Geometry: final body of the model. Coordinates: model frame, mm. A direction names the side the tool comes from. Give positions to 0.01 mm unless a question says otherwise; leave off trailing zeros. Order: outer loops, then holes, each group sorted by start corner. A loop starts at its lowest first (then second) coordinate and runs counter-clockwise, first axis right, second up. Notation, with made-up numbers: (-26, 75.5) -> (18, 75.5) arc R20 ccw to (18, 99.5) -> close; hole circle Ø9 at (-35, -34.5). An arc over 180 degrees is marked (long way). Write item = value, one per line.
```python
from build123d import *

# Parameters (mm, degrees)
F0_W     = 11
F0_H     = 30
F1_DEPTH = 24
F3_DEPTH = 11
F4_R     = 5
F4_R_2   = 2.5
F5_DEPTH = 41.001
F6_R     = 13
F7_R     = 5
F8_R     = 2


with BuildPart() as f1:
    # F0 (on Right) → F1 (new body, symmetric)
    with BuildSketch(Plane.YZ):
        with BuildLine():
            Line((-56, 0), (-30, 0))
            ThreePointArc((-30, 0), (-29.4730143031, 5.5983415304), (-27.9105714739, 11))
            Line((-27.9105714739, 11), (-56, 11))
            Line((-56, 11), (-56, 0))
        make_face()
        with BuildLine():
            Line((-30, 0), (-19, 0))
            ThreePointArc((-19, 0), (-18.1017503893, 5.7729223833), (-15.4919333848, 11))
            Line((-15.4919333848, 11), (-27.9105714739, 11))
            ThreePointArc((-27.9105714739, 11), (-29.4730143031, 5.5983415304), (-30, 0))
        make_face()
        with BuildLine():
            ThreePointArc((15.4919333848, 11), (18.1017503893, 5.7729223833), (19, 0))
            Line((19, 0), (30, 0))
            ThreePointArc((30, 0), (29.4730143031, 5.5983415304), (27.9105714739, 11))
            Line((27.9105714739, 11), (15.4919333848, 11))
        make_face()
        with BuildLine():
            ThreePointArc((-15.4919333848, 11), (0, 19), (15.4919333848, 11))
            Line((15.4919333848, 11), (27.9105714739, 11))
            ThreePointArc((27.9105714739, 11), (0, 30), (-27.9105714739, 11))
            Line((-27.9105714739, 11), (-15.4919333848, 11))
        make_face()
        with BuildLine():
            ThreePointArc((27.9105714739, 11), (29.4730143031, 5.5983415304), (30, 0))
            Line((30, 0), (51, 0))
            Line((51, 0), (51, 11))
            Line((51, 11), (40, 11))
            Line((40, 11), (27.9105714739, 11))
        make_face()
        with Locations((45.5, 26)):
            Rectangle(F0_W, F0_H)
    extrude(amount=F1_DEPTH, both=True)

    # F2 (on face) → F3 (cut, through all)
    with BuildSketch(Plane(origin=(0, 51, 0), x_dir=(-1, 0, 0), z_dir=(0, 1, 0))):
        with BuildLine():
            ThreePointArc((-6.5, 25), (0, 31.5), (6.5, 25))
            Line((6.5, 25), (6.5, 41))
            Line((6.5, 41), (-6.5, 41))
            Line((-6.5, 41), (-6.5, 25))
        make_face()
        with BuildLine():
            ThreePointArc((-6.5, 25), (0, 18.5), (6.5, 25))
            ThreePointArc((6.5, 25), (0, 31.5), (-6.5, 25))
        make_face()
    extrude(amount=-F3_DEPTH, mode=Mode.SUBTRACT)

    # F4 (on face) → F5 (cut, through all)
    with BuildSketch(Plane(origin=(0, 0, 0), x_dir=(1, 0, 0), z_dir=(0, 0, -1))):
        with Locations((11, 37.5)):
            Circle(F4_R)
        Circle(F4_R_2)
        with Locations((-11, 37.5)):
            Circle(F4_R)
    extrude(amount=-F5_DEPTH, mode=Mode.SUBTRACT)

    # F6
    f6_edges = [f1.edges().sort_by_distance(p)[0] for p in [
        (-24, -56, 5.5),
        (24, -56, 5.5),
    ]]
    fillet(f6_edges, radius=F6_R)

    # F7
    f7_edges = [f1.edges().sort_by_distance(p)[0] for p in [
        (-24, 45.5, 41),
        (24, 45.5, 41),
    ]]
    fillet(f7_edges, radius=F7_R)

    # F8
    f8_edges = [f1.edges().sort_by_distance(p)[0] for p in [
        (0, -27.910571, 11),
        (0, 27.910571, 11),
    ]]
    fillet(f8_edges, radius=F8_R)


solid = f1.part
```
1) Section query C-C (z = 16). Output: boundary loops of the cut face in (x, y).
Check sheet entries:
outline = (-24, -25.38) -> (24, -25.38) -> (24, -10.25) -> (-24, -10.25) -> close; (-24, 10.25) -> (24, 10.25) -> (24, 25.38) -> (-24, 25.38) -> close; (-24, 40) -> (24, 40) -> (24, 51) -> (-24, 51) -> close
2) Reachability of faces 4 (the face through (6, 40, 19)), 5 (the face through (6.5, 46, 33)), 6 (the face through (0, -42, 11)) from +Z, -Z, +X, -X, +Y, -Y: full face, straight path, thin tool, end or side. Return the list, or none.
Check sheet entries:
face_4 = +Z, +X, -X
face_5 = +Z, +Y
face_6 = +Z, +X, -X, -Y
3) Section query D-D (x = 12.5). Output: boundary loops of the cut face in (y, z), plus the area to 3 significant figures.
Check sheet entries:
outline = (-55.91, 0) -> (-42.27, 0) -> (-42.27, 11) -> (-55.91, 11) -> close; (-32.73, 0) -> (-19, 0) arc R19 cw to (19, 0) -> (51, 0) -> (51, 41) -> (40, 41) -> (40, 11) -> (29.24, 11) arc R2 cw to (27.41, 12.19) arc R30 ccw to (-27.41, 12.19) arc R2 cw to (-29.24, 11) -> (-32.73, 11) -> close
area = 1,600 mm²
4) First-contact query: P1, Ø10, axis at x = -0.5, y = -1, coming from the -Z side; P2, Ø3, axis at x = -18, z = 14, coming from the -Y side; P3, Ø11.5, axis at x = 11, y = -37.5, coming from the +Z side. Flat tips, straight axial feed; report the tip coordinate or a pass-through.
Check sheet entries:
P1 = 18.03
P2 = -27.27
P3 = 11
5) Section query A-A (y = -40.5). Output: boundary loops of the cut face in (x, z).
Check sheet entries:
outline = (-24, 0) -> (-15, 0) -> (-15, 11) -> (-24, 11) -> close; (-7, 0) -> (7, 0) -> (7, 11) -> (-7, 11) -> close; (15, 0) -> (24, 0) -> (24, 11) -> (15, 11) -> close
6) Section query B-B (y = 0). Output: boundary loops of the cut face in (x, z), plus the area to 3 significant figures.
Check sheet entries:
outline = (-24, 19) -> (-2.5, 19) -> (-2.5, 30) -> (-24, 30) -> close; (2.5, 19) -> (24, 19) -> (24, 30) -> (2.5, 30) -> close
area = 473 mm²
7) Mould query, pull axis Y, two halves, no side actions, for faces 1 (the face through (0, 51, 16)), 2 (the face through (-6.5, 46, 33)), 3 (the face through (-0.54, 2.44, 24.34)). Classes: +Y half, -Y half, draft (parallel to the pull), parting line (faces both ways), or undercut.
Check sheet entries:
face_1 = +Y half
face_2 = draft
face_3 = undercut
8) Line query: line 1 (X direction, y = -37, z = 2); line 2 (Y direction, x = -11, z = 7.5); line 3 (Y direction, x = 9.5, z = 36.5). Output: solid intervals per line, ascending. Write a range as from..to.
Check sheet entries:
line_1 = -24..-15.97, -6.03..6.03, 15.97..24
line_2 = -56..-42.5, -32.5..-17.46, 17.46..51
line_3 = 40..51
